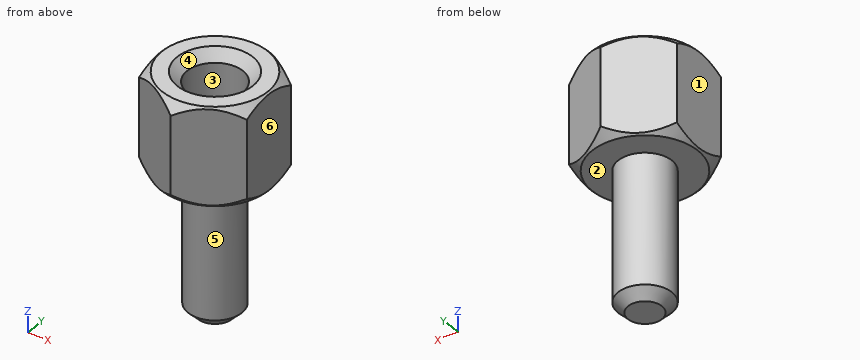
from build123d import *

# Parameters (mm, degrees)
RESSALTO_EXTRUS_O1_DEPTH = 4.9
ESBO_O10_R               = 1.35
RESSALTO_EXTRUS_O2_DEPTH = 7
ESBO_O11_R               = 1.4
CORTE_EXTRUS_O1_DEPTH    = 3.5
CHANFRO1_SIZE            = 0.5
CHANFRO2_SIZE            = 0.5


with BuildPart() as part:
    # Esboço1 → Ressalto-extrusão1 (new body)
    with BuildSketch(Plane.XY):
        Polygon((-2.727980022, 1.575), (-2.727980022, -1.575), (0, -3.15), (2.727980022, -1.575), (2.727980022, 1.575), (0, 3.15), align=None)
    extrude(amount=RESSALTO_EXTRUS_O1_DEPTH)

    # Esboço8 → Corte-Revolução1 (revolve, cut)
    with BuildSketch(Plane(origin=(0, 0, 0), x_dir=(0, 0, -1), z_dir=(1, 0, 0))):
        Polygon((-4.4, 3.15), (-4.9, 2.65), (-4.9, 3.15), align=None)
        Polygon((0, 3.15), (-0.5, 3.15), (0, 2.65), align=None)
    revolve(axis=Axis((0, 0, 0), (0, 0, 1)), mode=Mode.SUBTRACT)

    # Esboço10 → Ressalto-extrusão2 (add)
    with BuildSketch(Plane(origin=(0, 0, 0), x_dir=(-1, 0, 0), z_dir=(0, 0, -1))):
        with Locations(Location((0, 0, 0), (0, 0, 180))):
            Circle(ESBO_O10_R)
    extrude(amount=RESSALTO_EXTRUS_O2_DEPTH)

    # Esboço11 → Corte-extrusão1 (cut)
    with BuildSketch(Plane.XY.offset(4.9)):
        Circle(ESBO_O11_R)
    extrude(amount=-CORTE_EXTRUS_O1_DEPTH, mode=Mode.SUBTRACT)

    # Chanfro1
    chanfro1_edges = [part.edges().sort_by_distance(p)[0] for p in [
        (-1.4, 0, 4.9),
    ]]
    chamfer(chanfro1_edges, length=CHANFRO1_SIZE)

    # Chanfro2
    chanfro2_edges = [part.edges().sort_by_distance(p)[0] for p in [
        (-1.35, 0, -7),
    ]]
    chamfer(chanfro2_edges, length=CHANFRO2_SIZE)


solid = part.part
Here's how the part is built. I have some questions about the finished solid (model axes, mm). Face numbers are marked on the shaded views. A direction names the side the tool comes from. Coordinates: 2 decimals unless noted, no trailing zeros. Order: outer loops, then holes, each group sorted by start corner. A loop starts at its lowest first (then second) coordinate and runs counter-clockwise, first axis right, second up. Notation, with made-up numbers: (25, -21.75) - (36, -21.75) arc R15 cw to (36, -17.75) - close; hole circle Ø5 at (-10.75, 17). An arc over 180 degrees is marked (long way). Use CSV: the item, a comma, the result in double quotes. Start each with the question number.
1. Please list where these lines run through material, in increasing order: line 1 (Z direction, x = -0.85, y = -1.75); line 2 (Z direction, x = 0.7, y = 0); line 3 (Y direction, x = -1.8, z = 2.75). Write a range as from..to.
2. If we mould it in two halves opening along X, with no side actions, what happens to the marked faces 4, 5 and 6? For each: +X half, -X half, draft (parallel to the pull), parting line (faces both ways), or undercut.
3. For the marked faces 1, 2 and 3, which set-ups out of +Z, -Z, +X, -X, +Y, -Y let a thin tool reach every point of the face, with its end or its side?
4. Suppose I cut it at A-A on y = 0. List the corners of the cut face in (x, z) for me.
5. Suppose I cut it at B-B on z = -4.5. List the corners of the cut face in (x, y) for me.
6. I'm going to push flat-ended pins straight in: pin 1 (1 mm diameter, centred on x = 1, z = 0.5, fed in from -Y); pin 2 (3 mm diameter, centred on x = 0.5, y = -0.5, fed in from +Z); pin 3 (3 mm diameter, centred on y = -2.5, z = -5.5, fed in from +X). Where does each tip first touch, or does it pass through?
Output:
1,line 1,"z = 0..4.9"
1,line 2,"z = -7..1.4"
1,line 3,"y = -2.11..2.11"
2,face 4,"undercut"
2,face 5,"parting line"
2,face 6,"+X half"
3,face 1,"+Z, -Z, -X, +Y, -Y"
3,face 2,"-Z"
3,face 3,"+Z"
4,outline,"(-2.73, 0.08) - (-2.65, 0) - (-1.35, 0) - (-1.35, -6.5) - (-0.85, -7) - (0.85, -7) - (1.35, -6.5) - (1.35, 0) - (2.65, 0) - (2.73, 0.08) - (2.73, 4.82) - (2.65, 4.9) - (1.9, 4.9) - (1.4, 4.4) - (1.4, 1.4) - (-1.4, 1.4) - (-1.4, 4.4) - (-1.9, 4.9) - (-2.65, 4.9) - (-2.73, 4.82) - close"
5,outline,"circle Ø2.7 at (0, 0)"
6,pin 1,"stops at y = -2.86"
6,pin 2,"stops at z = 4.9"
6,pin 3,"stops at x = 0.91"
